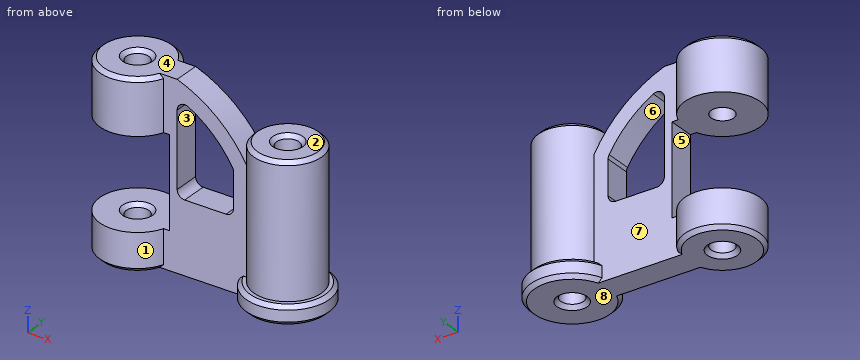
```python
from build123d import *

# Parameters (mm, degrees)
F0_R      = 25.4
F0_R_2    = 7.62
F1_DEPTH  = 123.19
F0_R_3    = 22.86
F3_DEPTH  = 101.6
F5_DEPTH  = 8.89
F6_W      = 60.96
F6_H      = 60.96
F7_DEPTH  = 50.8
F8_R      = 5.08
F9_SIZE   = 2.54
F10_R     = 27.94
F10_R_2   = 22.86
F11_DEPTH = 12.7
F12_SIZE  = 2.54


with BuildPart() as f1:
    # F0 (on Top) → F1 (new body)
    with BuildSketch(Plane.XY):
        Circle(F0_R)
        Circle(F0_R_2, mode=Mode.SUBTRACT)
    extrude(amount=F1_DEPTH)



with BuildPart() as f3:
    # F0 (on Top) → F3 (new body)
    with BuildSketch(Plane.XY):
        with Locations((101.6, 0)):
            Circle(F0_R_3)
        with Locations((101.6, 0)):
            Circle(F0_R_2, mode=Mode.SUBTRACT)
    extrude(amount=F3_DEPTH)


with BuildPart() as f1_1:
    add(f1.part)

    add(f3.part)  # F5 merges F3
    # F4 (on Front) → F5 (join, symmetric)
    with BuildSketch(Plane.XZ):
        with BuildLine():
            Line((20.32, 123.19), (20.32, 0))
            Line((20.32, 0), (81.28, 0))
            Line((81.28, 0), (81.28, 81.28))
            ThreePointArc((81.28, 81.28), (61.0468357955, 106.7222654615), (33.02, 123.19))
            Line((33.02, 123.19), (20.32, 123.19))
        make_face()
        with BuildLine():
            ThreePointArc((33.02, 111.6727406383), (54.9192892431, 98.053343988), (71.12, 77.988354443))
            Line((71.12, 77.988354443), (71.12, 48.1727406383))
            Line((71.12, 48.1727406383), (33.02, 48.1727406383))
            Line((33.02, 48.1727406383), (33.02, 111.6727406383))
        make_face(mode=Mode.SUBTRACT)
    extrude(amount=F5_DEPTH, both=True)

    # F6 (on Front) → F7 (cut, symmetric)
    with BuildSketch(Plane.XZ):
        with Locations((-2.54, 55.88)):
            Rectangle(F6_W, F6_H)
    extrude(amount=F7_DEPTH, both=True, mode=Mode.SUBTRACT)

    # F8
    f8_edges = [f1_1.edges().sort_by_distance(p)[0] for p in [
        (33.02, 0, 111.672741),
        (71.12, 0, 77.988354),
        (33.02, 0, 48.172741),
        (71.12, 0, 48.172741),
    ]]
    fillet(f8_edges, radius=F8_R)

    # F9
    f9_edges = [f1_1.edges().sort_by_distance(p)[0] for p in [
        (-7.62, 0, 123.19),
        (-25.4, 0, 123.19),
        (-7.62, 0, 25.4),
        (-7.62, 0, 0),
        (-25.4, 0, 0),
    ]]
    chamfer(f9_edges, length=F9_SIZE)

    # F10 (on Top) → F11 (join)
    with BuildSketch(Plane.XY):
        with Locations((101.6, 0)):
            Circle(F10_R)
        with Locations((101.6, 0)):
            Circle(F10_R_2, mode=Mode.SUBTRACT)
    extrude(amount=F11_DEPTH)

    # F12
    f12_edges = [f1_1.edges().sort_by_distance(p)[0] for p in [
        (93.98, 0, 0),
        (129.54, 0, 0),
        (93.98, 0, 101.6),
        (129.54, 0, 12.7),
        (78.74, 0, 101.6),
    ]]
    chamfer(f12_edges, length=F12_SIZE)


solid = f1_1.part
```
CAD build for the part. Positions are in the model's coordinates, mm. Face numbers are marked on the shaded views. A direction names the side the tool comes from. Coordinates: 2 decimals unless noted, no trailing zeros. Write each loop counter-clockwise with the first axis right and the second up, starting at its lowest first coordinate (ties: lowest second). Pieces come first, ordered by that corner, then holes. Notation, with made-up numbers: (-10, 14.5) -> (8, 14.5) arc R22 cw to (8, 34.5) -> close; hole circle Ø6 at (-15.5, -35). An arc over 180 degrees is marked (long way). Return JSON: item names as keys, results as strings. Group by question number.
Q1. Cut at A-A, the plane z = 64. Give the cut face in (x, y), then the cut area to 3 significant figures.
Q2. Which spindle directions (+Z, -Z, +X, -X, +Y, -Y) get a long thin tool onto all of the face, cutting with end or side? Do the marked faces 1, 2, 3, 4 and 5. Say none if no direction does.
Q3. Cut at B-B, the plane x = 0. Give the cut face in (y, z).
Q4. Flat gauge pins, fed straight in: pin 1 (9 mm diameter, centred on x = 0, y = 0, fed in from -Z); pin 2 (19.5 mm diameter, centred on y = 1, z = 61.5, fed in from -X); pin 3 (5 mm diameter, centred on x = 19.5, z = 21.5, fed in from -Y); pin 4 (1 mm diameter, centred on x = 112, y = 2.5, fed in from +Z). Where does each tip first touch, or does it go through?
Q5. Drill centre lines: line 1 (Z direction, x = 10, y = 12); line 2 (Y direction, x = 0, z = 98.5); line 3 (Y direction, x = 29.5, z = 8.5). Where is each one in solid material? Low to high.
Q6. Cut at C-C, the plane z = 18.5. Give the cut face in (x, y).
Q7. Cut at D-D, the plane z = 95. Give the cut face in (x, y), then the cut area to 3 significant figures.
Q8. Pull direction Z, two halves, no side cores. Call the marked faces 6, 7 and 8: released by +Z, released by -Z, zero draft, split by the parting line, or undercut.
Returned:
{
 "1": {"outline": "(27.94, -8.89) -> (33.02, -8.89) -> (33.02, 8.89) -> (27.94, 8.89) -> close; (71.12, -8.89) -> (80.54, -8.89) arc R22.86 ccw (long way) to (80.54, 8.89) -> (71.12, 8.89) -> close; hole circle Ø15.24 at (101.6, 0)", "area": "1,700 mm2"},
 "2": {"face 1": "+Z, -Z", "face 2": "+Z, +X, +Y, -Y", "face 3": "+Y, -Y", "face 4": "+Z, +X, -X, +Y, -Y", "face 5": "-X, +Y, -Y"},
 "3": {"outline": "(-25.4, 2.54) -> (-22.86, 0) -> (-10.16, 0) -> (-7.62, 2.54) -> (-7.62, 22.86) -> (-10.16, 25.4) -> (-25.4, 25.4) -> close; (-25.4, 86.36) -> (-7.62, 86.36) -> (-7.62, 120.65) -> (-10.16, 123.19) -> (-22.86, 123.19) -> (-25.4, 120.65) -> close; (7.62, 2.54) -> (10.16, 0) -> (22.86, 0) -> (25.4, 2.54) -> (25.4, 25.4) -> (10.16, 25.4) -> (7.62, 22.86) -> close; (7.62, 86.36) -> (25.4, 86.36) -> (25.4, 120.65) -> (22.86, 123.19) -> (10.16, 123.19) -> (7.62, 120.65) -> close"},
 "4": {"pin 1": "passes through", "pin 2": "stops at x = 27.94", "pin 3": "stops at y = -18.87", "pin 4": "stops at z = 101.6"},
 "5": {"line 1": "z = 0 to 25.4, 86.36 to 123.19", "line 2": "y = -25.4 to -7.62, 7.62 to 25.4", "line 3": "y = -8.89 to 8.89"},
 "6": {"outline": "(23.79, -8.89) -> (80.54, -8.89) arc R22.86 ccw (long way) to (80.54, 8.89) -> (23.79, 8.89) arc R25.4 ccw (long way) to start; hole circle Ø15.24 at (0, 0); hole circle Ø15.24 at (101.6, 0)"},
 "7": {"outline": "(23.79, -8.89) -> (33.02, -8.89) -> (33.02, 8.89) -> (23.79, 8.89) arc R25.4 ccw (long way) to start; (58.18, -8.89) -> (72.28, -8.89) -> (72.28, 8.89) -> (58.18, 8.89) -> close; circle Ø45.72 at (101.6, 0); hole circle Ø15.24 at (0, 0); hole circle Ø15.24 at (101.6, 0)", "area": "3,700 mm2"},
 "8": {"face 6": "undercut", "face 7": "zero draft", "face 8": "released by -Z"}
}
